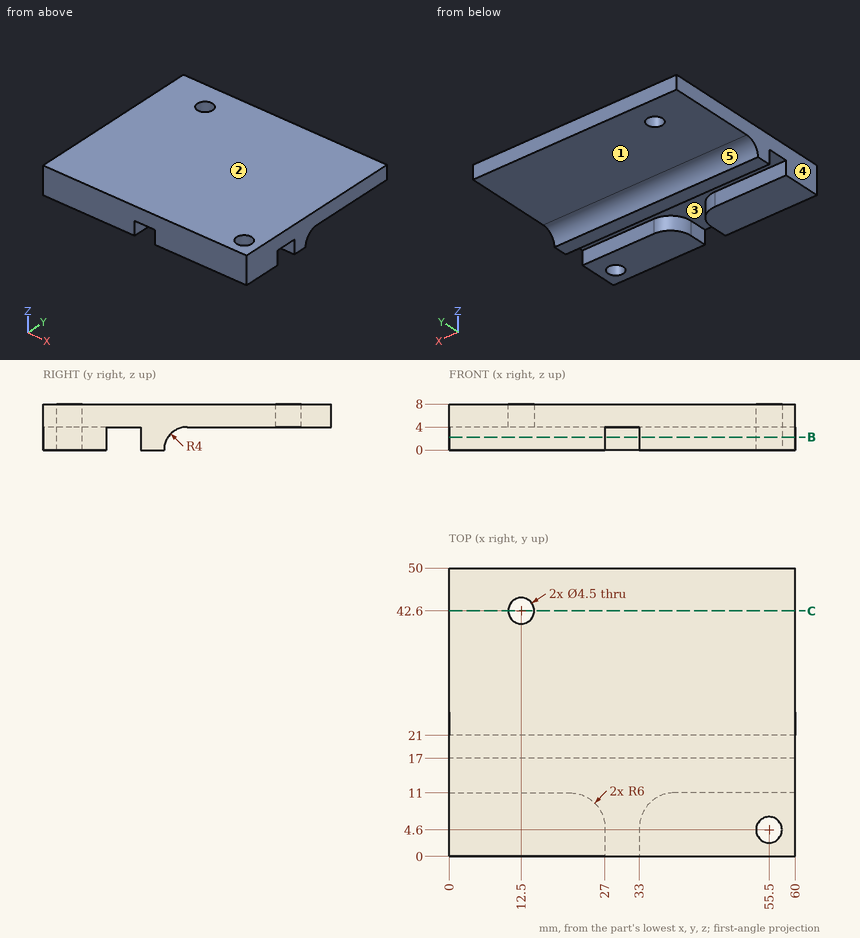
Study the drawing (mm; zero at the part's minimum x, y, z) and answer. A direction names the side the tool comes from. Round coordinates to 2 decimals unless told otherwise and drop trailing zeros. Order: outer loops, then holes, each group sorted by start corner. A loop starts at its lowest first (then second) coordinate and runs counter-clockwise, first axis right, second up. Notation, with made-up numbers: (71.25, 40.5) -> (85.25, 40.5) arc R18 cw to (85.25, 72.5) -> close; hole circle Ø9 at (47, -17.75). An arc over 180 degrees is marked (long way). Answer as CSV lines item,"result". Start each with the question number.
(1) Find the intervals of material crossed by probe 1 along Y at (x, z) = (12.5, 5.35); probe 2 along Z at (x, y) = (34.5, 26); probe 3 along Y at (x, z) = (55.5, 6.25), in increasing order. Write a range as from..to.
(2) The part is cut by section C-C (y = 42.6). Determine the outline of the cut face in (x, z).
(3) The part is cut by section B-B (z = 2.25). Determine the outline of the cut face in (x, y).
(4) For a pull along Y with two mould halves and no side action, classify the marked faces 3, 4 and 5 as +Y half, -Y half, draft (parallel to the pull), parting line (faces both ways), or undercut.
(5) Flat-ended cylindrical pins translate along their axes: pin 1 Ø3 at (y, z) = (1.5, 1.5) entering from -X; pin 2 Ø1.2 at (x, z) = (11, 2) entering from +Y; pin 3 Ø5 at (x, y) = (40, 24.5) entering from -Z; pin 4 Ø4.5 at (x, z) = (48.5, 1) entering from +Y. Find the tip coordinate at first contact, or state that the pin passes through.
(6) A tool of negligible diameter and unlimited length cuts with its end or side. For the marked faces 1 and 2, from which of +Z, -Z, +X, -X, +Y, -Y can it reach the whole face along a straight path? Write none if from no direction.
Evaluation:
1,probe 1,"0..40.35, 44.85..50"
1,probe 2,"4..8"
1,probe 3,"0..2.35, 6.85..50"
2,outline,"(0, 4) -> (10.25, 4) -> (10.25, 8) -> (0, 8) -> close; (14.75, 4) -> (60, 4) -> (60, 8) -> (14.75, 8) -> close"
3,outline,"(0, 0) -> (27, 0) -> (27, 5) arc R6 ccw to (21, 11) -> (0, 11) -> close; (0, 17) -> (60, 17) -> (60, 21.69) -> (0, 21.69) -> close; (33, 0) -> (60, 0) -> (60, 11) -> (39, 11) arc R6 ccw to (33, 5) -> close; hole circle Ø4.5 at (55.5, 4.6)"
4,face 3,"undercut"
4,face 4,"draft"
4,face 5,"+Y half"
5,pin 1,"x = 0"
5,pin 2,"y = 21.96"
5,pin 3,"z = 2.65"
5,pin 4,"y = 22.67"
6,face 1,"-Z, +X, -X, +Y"
6,face 2,"+Z, +X, -X, +Y, -Y"
